Verification items for the finished model (mm, model axes). Face numbers are marked on the shaded views. Round coordinates to 2 decimals unless told otherwise and drop trailing zeros. Write each loop counter-clockwise with the first axis right and the second up, starting at its lowest first coordinate (ties: lowest second). Pieces come first, ordered by that corner, then holes.
from build123d import *

# Parameters (mm, degrees)
SKETCH3_R          = 4
CUT_EXTRUDE1_DEPTH = 38.094473982


with BuildPart() as part:
    # Sketch2 → Revolve1 (revolve)
    with BuildSketch(Plane(origin=(0, 0, 0), x_dir=(0, 0, -1), z_dir=(1, 0, 0))):
        Polygon((0, -12), (0, 12), (20, 12), (20, 10), (12, 10), (12, 7.142857143), (18, 7.142857143), (18, 4.285714286), (12, 4.285714286), (12, 1.428571429), (18, 1.428571429), (18, -1.428571429), (12, -1.428571429), (12, -4.285714286), (18, -4.285714286), (18, -7.142857143), (12, -7.142857143), (12, -10), (20, -10), (20, -12), align=None)
    revolve(axis=Axis((0, -52.077930442, 0), (0, 1, 0)))

    # Sketch3 → Cut-Extrude1 (cut, through all)
    with BuildSketch(Plane(origin=(0, 12, 0), x_dir=(1, 0, 0), z_dir=(0, 1, 0))):
        with Locations(Location((0, 0, 0), (0, 0, 270))):
            Circle(SKETCH3_R)
    extrude(amount=-CUT_EXTRUDE1_DEPTH, mode=Mode.SUBTRACT)


solid = part.part
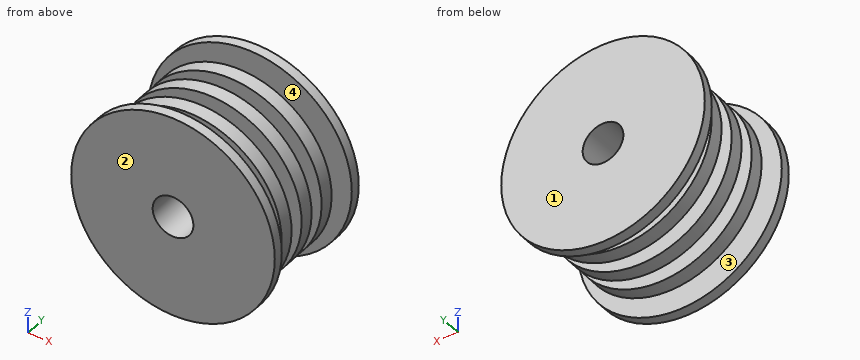
Q1. Sectioned sample at A-A (x = 16). Enter the section's corners in (y, z), plus the area to 3 significant figures.
Recorded:
outline: (-12, -12) - (-10, -12) - (-10, 12) - (-12, 12) - close; (-7.14, -8.25) - (-4.29, -8.25) - (-4.29, 8.25) - (-7.14, 8.25) - close; (-1.43, -8.25) - (1.43, -8.25) - (1.43, 8.25) - (-1.43, 8.25) - close; (4.29, -8.25) - (7.14, -8.25) - (7.14, 8.25) - (4.29, 8.25) - close; (10, -12) - (12, -12) - (12, 12) - (10, 12) - close
area: 237 mm2
Q2. Material ranges on line 1 along Y through (x, z) = (-14.5, -5.5); line 2 along X through (y, z) = (-5.5, 0); line 3 along Y through (x, z) = (18, 2), recorded low to high.
Recorded:
line 1: y = -12 to -10, -7.14 to -4.29, -1.43 to 1.43, 4.29 to 7.14, 10 to 12
line 2: x = -18 to -4, 4 to 18
line 3: y = -12 to -10, 10 to 12
Q3. Release check for a two-part mould opening along Y. For the marked faces 1, 2, 3 and 4 record: released by +Y, released by -Y, zero draft, split by the parting line, or undercut.
Recorded:
face 1: released by +Y
face 2: released by -Y
face 3: undercut
face 4: undercut
Q4. Depth check by flat-ended pin: P1, Ø6.5, axis at x = 0, z = 0, coming from the -Y side; P2, Ø3, axis at x = -7.5, y = -8, coming from the -Z side; P3, Ø1.5, axis at x = -6, y = -6, coming from the +Z side; P4, Ø8, axis at x = 16, y = -1, coming from the -Z side. Enter the tip coordinate at first touch or a pass-through.
Recorded:
P1: passes through
P2: stops at z = -16.87
P3: stops at z = 17.22
P4: stops at z = -13.42
Q5. Sectioned sample at B-B (y = -5). Enter the section's corners in (x, z).
Recorded:
outline: circle Ø36 at (0, 0); hole circle Ø8 at (0, 0)
Q6. Sectioned sample at C-C (x = -15). Enter the section's corners in (y, z).
Recorded:
outline: (-12, -13.23) - (-10, -13.23) - (-10, 13.23) - (-12, 13.23) - close; (-7.14, -9.95) - (-4.29, -9.95) - (-4.29, 9.95) - (-7.14, 9.95) - close; (-1.43, -9.95) - (1.43, -9.95) - (1.43, 9.95) - (-1.43, 9.95) - close; (4.29, -9.95) - (7.14, -9.95) - (7.14, 9.95) - (4.29, 9.95) - close; (10, -13.23) - (12, -13.23) - (12, 13.23) - (10, 13.23) - close
